Input: part model. Units: mm. Frame: model coordinates. Give positions to 0.01 mm unless a question says otherwise; leave off trailing zeros. Loops run counter-clockwise (first coordinate to the right, second up) from the corner with the lowest first, then second, coordinate; pieces in that order, holes last. Notation, with made-up numbers: M -3,-4 L 15,-4 A32 ccw 15,30 Z; hole C 55.5,46.25 d4. An arc over 180 degrees is marked long. Answer as a JSON object with one key per item and string values. Group by question number.
1) Section query D-D on y = 118.5. Return loops of the section in (x, z), plus the area to 3 significant figures.
2) Draft query along X for faces 1 (the cylindrical face through (-107.287, 21.139, 6.261)), 2 (the flat face through (10.922, 127.469, 6.439)), 3 (the flat face through (-15.852, 20.776, 6.261)). Return one class per face: +X half, -X half, draft (parallel to the pull), parting line (faces both ways), or undercut.
3) First-contact query: P1, Ø5, axis at y = 59.5, z = 6, coming from the -X side; P2, Ø3, axis at y = 147, z = 5.5, coming from the -X side; P3, Ø4, axis at y = 66, z = 4.5, coming from the -X side; P4, Ø9.5, axis at x = -42.71, y = 45.26, coming from the +Z side. Flat tips, straight axial feed; report the tip coordinate or a pass-through.
4) Section query B-B on y = 87. Return loops of the section in (x, z), plus the area to 3 significant figures.
5) Section query C-C on y = -3. Return loops of the section in (x, z).
6) Section query A-A on x = -78.5. Return loops of the section in (y, z).
7) Ray query, L1, parallel to X at y = 106.5, z = 10; L2, parallel to Y at x = 6, z = 2.25; L3, parallel to Y at x = -85.5, z = 11.25. Return the intervals inside material, ascending.
from build123d import *

# Parameters (mm, degrees)
BOSS_EXTRUDE1_DEPTH = 12.7
SKETCH2_R           = 7.9375
CUT_EXTRUDE1_DEPTH  = 25.4
CUT_EXTRUDE2_DEPTH  = 25.4
CUT_EXTRUDE3_DEPTH  = 25.4
CUT_EXTRUDE4_DEPTH  = 25.4
CUT_EXTRUDE5_DEPTH  = 25.4


with BuildPart() as part:
    # Sketch1 → Boss-Extrude1 (new body)
    with BuildSketch(Plane.XY):
        with BuildLine():
            Line((29.67833379, 155.20549492), (-42.163715178, 83.363445951))
            Line((-42.163715178, 83.363445951), (-118.363715178, 83.363445951))
            ThreePointArc((-118.363715178, 83.363445951), (-106.853658004, 20.335826766), (-60.124227421, -23.497066291))
            Line((-60.124227421, -23.497066291), (29.67833379, 66.30549492))
            Line((29.67833379, 66.30549492), (105.87833379, 66.30549492))
            Line((105.87833379, 66.30549492), (105.87833379, 155.20549492))
            Line((105.87833379, 155.20549492), (29.67833379, 155.20549492))
        make_face()
    extrude(amount=BOSS_EXTRUDE1_DEPTH)

    # Sketch2 → Cut-Extrude1 (cut)
    with BuildSketch(Plane.XY.offset(12.7)):
        with Locations((-42.71166621, 45.263445951)):
            Circle(SKETCH2_R)
    extrude(amount=-CUT_EXTRUDE1_DEPTH, mode=Mode.SUBTRACT)

    # Sketch3 → Cut-Extrude2 (cut)
    with BuildSketch(Plane.XY.offset(12.7)):
        Polygon((93.17833379, 143.77549492), (67.77833379, 114.880205391), (42.37833379, 143.77549492), (42.37833379, 150.12549492), (93.17833379, 150.12549492), align=None)
        Polygon((97.62333379, 139.96549492), (71.946691953, 110.75549492), (97.62333379, 81.54549492), (100.79833379, 81.54549492), (100.79833379, 139.96549492), align=None)
        Polygon((34.75833379, 139.96549492), (37.93333379, 139.96549492), (63.609975627, 110.75549492), (37.93333379, 81.54549492), (34.75833379, 81.54549492), align=None)
        Polygon((42.37833379, 71.38549492), (42.37833379, 77.73549492), (67.77833379, 106.630784448), (93.17833379, 77.73549492), (93.17833379, 71.38549492), align=None)
    extrude(amount=-CUT_EXTRUDE2_DEPTH, mode=Mode.SUBTRACT)

    # Sketch4 → Cut-Extrude3 (cut)
    with BuildSketch(Plane.XY.offset(12.7)):
        Polygon((-7.061410089, 109.48549492), (28.40833379, 74.015751041), (28.40833379, 144.955238799), align=None)
        Polygon((23.91820573, 69.52562298), (-11.551538149, 34.055879101), (-11.551538149, 104.995366859), align=None)
        Polygon((-17.901538149, 98.645366859), (-47.021282028, 69.52562298), (-17.901538149, 40.405879101), align=None)
    extrude(amount=-CUT_EXTRUDE3_DEPTH, mode=Mode.SUBTRACT)

    # Sketch5 → Cut-Extrude4 (cut)
    with BuildSketch(Plane.XY.offset(12.7)):
        with BuildLine():
            Line((-29.010735503, 42.534820334), (-16.04166621, 29.565751041))
            Line((-16.04166621, 29.565751041), (-29.512050392, 16.095366859))
            Line((-29.512050392, 16.095366859), (-44.879327107, 31.462643575))
            ThreePointArc((-44.879327107, 31.462643575), (-34.717771497, 33.806633684), (-29.010735503, 42.534820334))
        make_face()
        with BuildLine():
            Line((-44.434025607, 59.126864653), (-62.320606906, 77.013445951))
            Line((-62.320606906, 77.013445951), (-89.539393744, 77.013445951))
            Line((-89.539393744, 77.013445951), (-56.633788009, 44.107840216))
            ThreePointArc((-56.633788009, 44.107840216), (-53.555107626, 54.071435408), (-44.434025607, 59.126864653))
        make_face()
    extrude(amount=-CUT_EXTRUDE4_DEPTH, mode=Mode.SUBTRACT)

    # Sketch6 → Cut-Extrude5 (cut)
    with BuildSketch(Plane.XY.offset(12.7)):
        with BuildLine():
            Line((-56.837225548, -11.229808297), (-33.556810582, 12.050606669))
            Line((-33.556810582, 12.050606669), (-98.519649865, 77.013445951))
            Line((-98.519649865, 77.013445951), (-105.663715178, 77.013445951))
            ThreePointArc((-105.663715178, 77.013445951), (-94.97435542, 25.298160398), (-56.837225548, -11.229808297))
        make_face()
    extrude(amount=-CUT_EXTRUDE5_DEPTH, mode=Mode.SUBTRACT)


solid = part.part
Output:
{
 "1": {"outline": "M -7.03,0 L 1.95,0 L 1.95,12.7 L -7.03,12.7 Z; M 28.41,0 L 34.76,0 L 34.76,12.7 L 28.41,12.7 Z; M 56.8,0 L 64.6,0 L 64.6,12.7 L 56.8,12.7 Z; M 70.96,0 L 78.75,0 L 78.75,12.7 L 70.96,12.7 Z; M 100.8,0 L 105.88,0 L 105.88,12.7 L 100.8,12.7 Z", "area": "457 mm^2"},
 "2": {"face 1": "-X half", "face 2": "undercut", "face 3": "+X half"},
 "3": {"P1": "stops at x = -119.07", "P2": "stops at x = 19.97", "P3": "stops at x = -119.32", "P4": "passes through"},
 "4": {"outline": "M -38.53,0 L -29.55,0 L -29.55,12.7 L -38.53,12.7 Z; M -17.9,0 L -11.55,0 L -11.55,12.7 L -17.9,12.7 Z; M 6.44,0 L 15.42,0 L 15.42,12.7 L 6.44,12.7 Z; M 28.41,0 L 34.76,0 L 34.76,12.7 L 28.41,12.7 Z; M 42.73,0 L 50.52,0 L 50.52,12.7 L 42.73,12.7 Z; M 85.03,0 L 92.83,0 L 92.83,12.7 L 85.03,12.7 Z; M 100.8,0 L 105.88,0 L 105.88,12.7 L 100.8,12.7 Z", "area": "652 mm^2"},
 "5": {"outline": "M -89.41,0 L -70.24,0 L -70.24,12.7 L -89.41,12.7 Z; M -48.61,0 L -39.63,0 L -39.63,12.7 L -48.61,12.7 Z"},
 "6": {"outline": "M -12.48,0 L 3.96,0 L 3.96,12.7 L -12.48,12.7 Z; M 56.99,0 L 65.97,0 L 65.97,12.7 L 56.99,12.7 Z; M 77.01,0 L 83.36,0 L 83.36,12.7 L 77.01,12.7 Z"},
 "7": {"L1": "x = -19.03 to -4.08, 28.41 to 34.76, 59.87 to 67.66, 67.89 to 75.69, 100.8 to 105.88", "L2": "y = 42.63 to 51.61, 87.44 to 96.42, 122.55 to 131.53", "L3": "y = -6.72 to 11.45, 63.99 to 72.97, 77.01 to 83.36"}
}
